Geometry check sheet. Reference: the model listing, model coordinates, mm. Face numbers are marked on the shaded views. A direction names the side the tool comes from. Coordinates: 2 decimals unless noted, no trailing zeros. Order: outer loops, then holes, each group sorted by start corner. A loop starts at its lowest first (then second) coordinate and runs counter-clockwise, first axis right, second up. Notation, with made-up numbers: (71, 27) - (119, 27) arc R29 cw to (119, 56) - close; hole circle Ø3 at (-23.75, 24.25). An arc over 180 degrees is marked (long way). Return JSON: item names as keys, results as strings. Group by question number.
Item 1: Gauge pin test, flat ends, axial feed: pin 1 (5 mm diameter, centred on x = -4, y = 228.5, fed in from -Z); pin 2 (6 mm diameter, centred on x = 0, z = -18.75, fed in from -Y); pin 3 (1.5 mm diameter, centred on y = 283.5, z = -26, fed in from +X); pin 4 (2 mm diameter, centred on x = 50, z = -24.5, fed in from +Y). Record the tip position at first contact, or that the pin passes through.
Item 2: Scan lines: probe 1 along Z at (x, y) = (0, 191.5); probe 2 along Z at (x, y) = (0, 320); probe 3 along Z at (x, y) = (72.5, -40). Record each from-to range of solid material in increasing order.
Item 3: Draft check along X on the marked faces 3, 4 and 5. Enter one of: pulls with the +X half, pulls with the -X half, needs draft (parallel to the pull), parting line crosses it, or undercut.
Item 4: Tool access check on the marked faces 1 and 2. Record the directions out of +Z, -Z, +X, -X, +Y, -Y that give a thin tool (end or side, any length) a straight path to the whole face; none if there is none.
Item 5: Section check C-C on x = 37. Enter the section's corners in (y, z), then the cut area to 3 significant figures.
Item 6: Section check D-D on z = 98. Enter the section's corners in (x, y).
Item 7: Section check A-A on x = -10. Enter the section's corners in (y, z).
Item 8: Section check B-B on z = 7. Enter the section's corners in (x, y).
from build123d import *

# Parameters (mm, degrees)
SKETCH1_R           = 28.1
BOSS_EXTRUDE1_DEPTH = 350
SKETCH2_R           = 18.6
CUT_EXTRUDE1_DEPTH  = 58.8
SKETCH3_W           = 222.683092022
SKETCH3_H           = 364.2827524
BOSS_EXTRUDE2_DEPTH = 58.8
SKETCH4_W           = 207.917403516
SKETCH4_H           = 348.54429772
CUT_EXTRUDE2_DEPTH  = 48.8
SKETCH5_R           = 16.1
CUT_EXTRUDE3_DEPTH  = 350
SKETCH6_R           = 3.75
CUT_EXTRUDE5_DEPTH  = 400


with BuildPart() as part:
    # Sketch1 → Boss-Extrude1 (new body)
    with BuildSketch(Plane(origin=(0, 0, 0), x_dir=(1, 0, 0), z_dir=(0, 1, 0))):
        Circle(SKETCH1_R)
    extrude(amount=BOSS_EXTRUDE1_DEPTH)

    # Sketch2 → Cut-Extrude1 (cut)
    with BuildSketch(Plane(origin=(0, 350, 0), x_dir=(1, 0, 0), z_dir=(0, 1, 0))):
        with Locations((0, -7)):
            Circle(SKETCH2_R)
    extrude(amount=-CUT_EXTRUDE1_DEPTH, mode=Mode.SUBTRACT)

    # Sketch3 → Boss-Extrude2 (add)
    with BuildSketch(Plane(origin=(0, 0, 0), x_dir=(-1, 0, 0), z_dir=(0, -1, 0))):
        Rectangle(SKETCH3_W, SKETCH3_H)
    extrude(amount=BOSS_EXTRUDE2_DEPTH)

    # Sketch4 → Cut-Extrude2 (cut)
    with BuildSketch(Plane(origin=(0, -58.8, 0), x_dir=(-1, 0, 0), z_dir=(0, -1, 0))):
        Rectangle(SKETCH4_W, SKETCH4_H)
    extrude(amount=-CUT_EXTRUDE2_DEPTH, mode=Mode.SUBTRACT)

    # Sketch5 → Cut-Extrude3 (cut)
    with BuildSketch(Plane(origin=(0, 291.2, 0), x_dir=(1, 0, 0), z_dir=(0, 1, 0))):
        with Locations((0, -7)):
            Circle(SKETCH5_R)
    extrude(amount=-CUT_EXTRUDE3_DEPTH, mode=Mode.SUBTRACT)

    # Sketch6 → Cut-Extrude5 (cut)
    with BuildSketch(Plane(origin=(0, 350, 0), x_dir=(1, 0, 0), z_dir=(0, 1, 0))):
        with Locations((0, 18.75)):
            Circle(SKETCH6_R)
    extrude(amount=-CUT_EXTRUDE5_DEPTH, mode=Mode.SUBTRACT)


solid = part.part
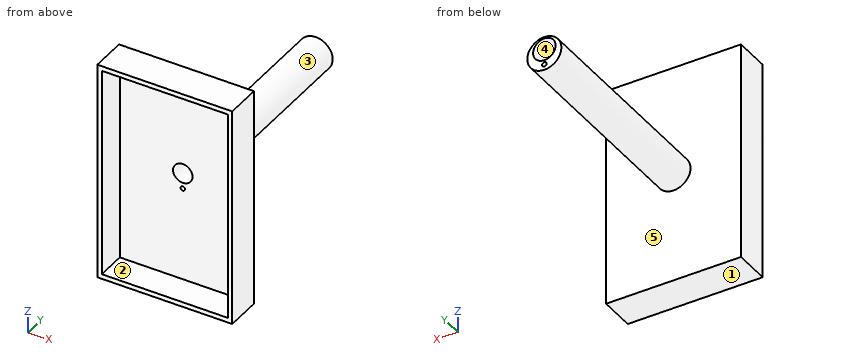
Computed:
{
 "1": {"pin 1": "stops at z = -28.06", "pin 2": "passes through", "pin 3": "stops at x = 12.33", "pin 4": "stops at y = 0"},
 "2": {"probe 1": "z = -28.1 to -22.5, -15 to -9.1, 23.1 to 28.1", "probe 2": "z = -28.1 to -22.5, -15 to -11.6, 25.6 to 28.1", "probe 3": "z = -182.14 to -174.27, 174.27 to 182.14"},
 "3": {"face 3": "parting line crosses it", "face 4": "undercut", "face 5": "needs draft"},
 "4": {"face 1": "-Z, +X, -X, +Y, -Y", "face 2": "-Y"},
 "5": {"outline": "(-58.8, -182.14) - (0, -182.14) - (0, 182.14) - (-58.8, 182.14) - (-58.8, 174.27) - (-10, 174.27) - (-10, -174.27) - (-58.8, -174.27) - close", "area": "4,410 mm²"},
 "6": {"outline": "(-111.34, -58.8) - (-103.96, -58.8) - (-103.96, -10) - (103.96, -10) - (103.96, -58.8) - (111.34, -58.8) - (111.34, 0) - (-111.34, 0) - close"},
 "7": {"outline": "(-58.8, -182.14) - (0, -182.14) - (0, -26.26) - (350, -26.26) - (350, -8.68) - (291.2, -8.68) - (291.2, -5.62) - (-10, -5.62) - (-10, -174.27) - (-58.8, -174.27) - close; (-58.8, 174.27) - (-10, 174.27) - (-10, 19.62) - (291.2, 19.62) - (291.2, 22.68) - (350, 22.68) - (350, 26.26) - (0, 26.26) - (0, 182.14) - (-58.8, 182.14) - close"},
 "8": {"outline": "(-111.34, -58.8) - (-103.96, -58.8) - (-103.96, -10) - (-16.1, -10) - (-16.1, 291.2) - (-18.6, 291.2) - (-18.6, 350) - (-27.21, 350) - (-27.21, 0) - (-111.34, 0) - close; (16.1, -10) - (103.96, -10) - (103.96, -58.8) - (111.34, -58.8) - (111.34, 0) - (27.21, 0) - (27.21, 350) - (18.6, 350) - (18.6, 291.2) - (16.1, 291.2) - close"}
}
